from build123d import *

# Parameters (mm, degrees)
SKETCH1_R           = 16.5
BOSS_EXTRUDE1_DEPTH = 6
SKETCH4_R           = 5
SKETCH6_R           = 3.85
CUT_EXTRUDE1_DEPTH  = 7.5
SKETCH7_R           = 1.75
CUT_EXTRUDE2_DEPTH  = 28.21212977
SKETCH9_R           = 2.25
CUT_EXTRUDE3_DEPTH  = 25.834452009
FILLET1_R           = 2
CUT_EXTRUDE4_DEPTH  = 2.5


with BuildPart() as part:
    # Sketch1 → Boss-Extrude1 (new body)
    with BuildSketch(Plane(origin=(0, 0, 0), x_dir=(1, 0, 0), z_dir=(0, 1, 0))):
        with Locations(Location((0, 0, 0), (0, 0, 270))):
            Circle(SKETCH1_R)
    extrude(amount=-BOSS_EXTRUDE1_DEPTH)

    # Sketch4 → section 0 of loft1
    with BuildSketch(Plane(origin=(0, 8, 0), x_dir=(1, 0, 0), z_dir=(0, 1, 0)), mode=Mode.PRIVATE) as loft1_s0:
        Circle(SKETCH4_R)
    # loft up to a face of the part (loft1)
    loft([loft1_s0.sketch, part.faces().sort_by_distance((0, 0, 0))[0]])

    # Sketch6 → Cut-Extrude1 (cut)
    with BuildSketch(Plane(origin=(0, 8, 0), x_dir=(1, 0, 0), z_dir=(0, 1, 0))):
        with Locations(Location((0, 11.5, 0), (0, 0, 270))):
            Circle(SKETCH6_R)
        with Locations(Location((11.5, 0, 0), (0, 0, 270))):
            Circle(SKETCH6_R)
        with Locations(Location((0, -11.5, 0), (0, 0, 270))):
            Circle(SKETCH6_R)
        with Locations(Location((-11.5, 0, 0), (0, 0, 270))):
            Circle(SKETCH6_R)
    extrude(amount=-CUT_EXTRUDE1_DEPTH, mode=Mode.SUBTRACT)

    # Sketch7 → Cut-Extrude2 (cut, through all)
    with BuildSketch(Plane(origin=(0, 8, 0), x_dir=(1, 0, 0), z_dir=(0, 1, 0))):
        with Locations(Location((0, 0, 0), (0, 0, 270))):
            Circle(SKETCH7_R)
    extrude(amount=-CUT_EXTRUDE2_DEPTH, mode=Mode.SUBTRACT)

    # Sketch9 → Cut-Extrude3 (cut, through all)
    with BuildSketch(Plane(origin=(0, 2.5, 0), x_dir=(1, 0, 0), z_dir=(0, 1, 0))):
        with Locations(Location((0, 11.5, 0), (0, 0, 270))):
            Circle(SKETCH9_R)
        with Locations(Location((11.5, 0, 0), (0, 0, 270))):
            Circle(SKETCH9_R)
        with Locations(Location((0, -11.5, 0), (0, 0, 270))):
            Circle(SKETCH9_R)
        with Locations(Location((-11.5, 0, 0), (0, 0, 270))):
            Circle(SKETCH9_R)
    extrude(amount=-CUT_EXTRUDE3_DEPTH, mode=Mode.SUBTRACT)

    # Fillet1
    fillet1_edges = [part.edges().sort_by_distance(p)[0] for p in [
        (11.66726189, 0, 11.66726189),
    ]]
    fillet(fillet1_edges, radius=FILLET1_R)

    # Sketch10 → Cut-Extrude4 (cut)
    with BuildSketch(Plane.XZ.offset(6)):
        Polygon((1.732050808, -3), (3.464101615, 0), (1.732050808, 3), (-1.732050808, 3), (-3.464101615, 0), (-1.732050808, -3), align=None)
    extrude(amount=-CUT_EXTRUDE4_DEPTH, mode=Mode.SUBTRACT)


solid = part.part
Input: part model. Units: mm. Frame: model coordinates. A direction names the side the tool comes from. Give positions to 0.01 mm unless a question says otherwise; leave off trailing zeros. Loops run counter-clockwise (first coordinate to the right, second up) from the corner with the lowest first, then second, coordinate; pieces in that order, holes last. Notation, with made-up numbers: (12, 11) -> (21, 11) arc R18 ccw to (21, 21) -> close; hole circle Ø3 at (10.25, -15). An arc over 180 degrees is marked (long way). Answer as a JSON object with one key per item and string values. Group by question number.
Item 1: Line query: probe 1 along X at (y, z) = (-2, 0); probe 2 along Z at (x, y) = (-10.5, -0.75); probe 3 along X at (y, z) = (-1.5, -11.5). Output: solid intervals per line, ascending.
Item 2: Cut plane A-A, the plane y = -4.25. Return the cut outline in (x, z).
Item 3: Cut plane B-B, the plane y = 4. Return the cut outline in (x, z).
Item 4: Reachability of faces 1 (the flat face through (-2, 0.5, 13)), 2 (the flat face through (0, -5, -3)), 3 (the cylindrical face through (-1.71, 2.33, -0.38)) from +Z, -Z, +X, -X, +Y, -Y: full face, straight path, thin tool, end or side. Return the list, or none.
Item 5: Pull-direction query (Z, two-part tool) for faces 4 (the flat face through (-2.6, -4.8, -1.5)), 5 (the flat face through (2, 8, 0)), 6 (the cylindrical face through (4.956, -3.487, 15.738)); classes: released by +Z, released by -Z, zero draft, split by the parting line, or undercut.
Item 6: Cut plane C-C, the plane y = -2. Return the cut outline in (x, z), and give its area (3 significant figures).
Item 7: Pin query (flat end, axial travel): P1, Ø2, axis at x = -12, y = 0.5, coming from the -Z side; P2, Ø6, axis at x = 0, z = -11.5, coming from the +Y side; P3, Ø5, axis at x = -12, y = 0, coming from the +Z side. Return the tip coordinate at first contact, or that it passes through.
Checks:
{
 "1": {"probe 1": "x = -16.5 to -13.75, -9.25 to -1.75, 1.75 to 9.25, 13.75 to 16.5", "probe 2": "z = -12.7 to -2.02, 2.02 to 12.7", "probe 3": "x = -11.83 to -2.25, 2.25 to 11.83"},
 "2": {"outline": "circle Ø33 at (0, 0); hole circle Ø4.5 at (-11.5, 0); hole (-3.46, 0) -> (-1.73, -3) -> (1.73, -3) -> (3.46, 0) -> (1.73, 3) -> (-1.73, 3) -> close; hole circle Ø4.5 at (0, -11.5); hole circle Ø4.5 at (0, 11.5); hole circle Ø4.5 at (11.5, 0)"},
 "3": {"outline": "(-10.13, -3.6) arc R10.75 ccw to (-3.6, -10.13) arc R3.85 cw to (3.6, -10.13) arc R10.75 ccw to (10.13, -3.6) arc R3.85 cw to (10.13, 3.6) arc R10.75 ccw to (3.6, 10.13) arc R3.85 cw to (-3.6, 10.13) arc R10.75 ccw to (-10.13, 3.6) arc R3.85 cw to start; hole circle Ø3.5 at (0, 0)"},
 "4": {"face 1": "+Y", "face 2": "-Y", "face 3": "+Y, -Y"},
 "5": {"face 4": "undercut", "face 5": "zero draft", "face 6": "split by the parting line"},
 "6": {"outline": "circle Ø33 at (0, 0); hole circle Ø4.5 at (-11.5, 0); hole circle Ø4.5 at (0, -11.5); hole circle Ø4.5 at (0, 11.5); hole circle Ø3.5 at (0, 0); hole circle Ø4.5 at (11.5, 0)", "area": "782 mm²"},
 "7": {"P1": "stops at z = -11.79", "P2": "stops at y = 0.5", "P3": "stops at z = 13.38"}
}
